from build123d import *

# Parameters (mm, degrees)
BOSS_EXTRUDE1_DEPTH = 50
SKETCH2_R           = 22.5
BOSS_EXTRUDE2_DEPTH = 20
SKETCH3_R           = 22.5
BOSS_EXTRUDE3_DEPTH = 20
CHAMFER2_SIZE       = 2


with BuildPart() as part:
    # Sketch1 → Boss-Extrude1 (new body)
    with BuildSketch(Plane.XY):
        Polygon((0, 275), (0, 0), (275, 0), (275, 15), (15, 15), (15, 275), align=None)
    extrude(amount=BOSS_EXTRUDE1_DEPTH)

    # Sketch2 → Boss-Extrude2 (add)
    with BuildSketch(Plane(origin=(0, 15, 0), x_dir=(1, 0, 0), z_dir=(0, 1, 0))):
        with Locations((145, -25)):
            Circle(SKETCH2_R)
    extrude(amount=BOSS_EXTRUDE2_DEPTH)

    # Sketch3 → Boss-Extrude3 (add)
    with BuildSketch(Plane(origin=(15, 0, 0), x_dir=(0, 0, -1), z_dir=(1, 0, 0))):
        with Locations(Location((-25, 145, 0), (0, 0, 180))):
            Circle(SKETCH3_R)
    extrude(amount=BOSS_EXTRUDE3_DEPTH)

    # Chamfer2
    chamfer2_edges = [part.edges().sort_by_distance(p)[0] for p in [
        (0, 0, 25),
        (0, 275, 25),
        (0, 137.5, 0),
        (0, 137.5, 50),
    ]]
    chamfer(chamfer2_edges, length=CHAMFER2_SIZE)


solid = part.part
CAD build for the part. Positions are in the model's coordinates, mm. A direction names the side the tool comes from. Give positions to 0.01 mm unless a question says otherwise; leave off trailing zeros. Loops run counter-clockwise (first coordinate to the right, second up) from the corner with the lowest first, then second, coordinate; pieces in that order, holes last. Notation, with made-up numbers: M -31,-4 L 14,-4 A30 ccw 14,35 Z; hole C 85.25,38 d11. An arc over 180 degrees is marked long. One line per question, with ' | ' between items. Start each with the question number.
1. Saw through at C-C on y = 145. Give the cut face in (x, z), plus the area to 3 significant figures.
2. Saw through at A-A on x = 145. Give the cut face in (y, z), plus the area to 3 significant figures.
3. 3-axis set-ups, long thin cutter, end or side, ignore diameter. For faces 1 (the face through (137, 0, 25)), 2 (the face through (166.46, 24.86, 18.24)), 3 (the face through (35, 145, 25)): which of +Z, -Z, +X, -X, +Y, -Y reach the whole face in a straight line?
4. Flat gauge pins, fed straight in: pin 1 (13.5 mm diameter, centred on x = 135.5, z = 19.5, fed in from +Y); pin 2 (22.5 mm diameter, centred on y = 137.5, z = 23.5, fed in from +X); pin 3 (12 mm diameter, centred on y = 74.5, z = 45, fed in from +X). Where does each tip first touch, or does it go through?
5. Two-plate mould, pull along X, no slides. Class faces 4 (the face through (147, 15, 2)), 5 (the face through (24.86, 122.69, 22.07)), 6 (the face through (0, 139, 25)): pulls with the +X half, pulls with the -X half, needs draft (parallel to the pull), parting line crosses it, or undercut.
6. Saw through at D-D on z = 6.5. Give the cut face in (x, y).
7. Probe L1, parallel to X at y = 167, z = 30.5; L2, parallel to Y at x = 160.5, z = 36. List the from-to ranges inside material, lowest first. Write a range as from..to.
8. Saw through at B-B on z = 25. Give the cut face in (x, y), plus the area to 3 significant figures.
Result sheet:
1) outline: M 0,2 L 2,0 L 15,0 L 15,2.5 L 35,2.5 L 35,47.5 L 15,47.5 L 15,50 L 2,50 L 0,48 Z | area: 1,650 mm^2
2) outline: M 0,0 L 15,0 L 15,2.5 L 35,2.5 L 35,47.5 L 15,47.5 L 15,50 L 0,50 Z | area: 1,650 mm^2
3) face 1: +Z, -Z, +X, -X, -Y | face 2: +Y | face 3: +Z, -Z, +X, +Y
4) pin 1: stops at y = 35 | pin 2: stops at x = 35 | pin 3: stops at x = 15
5) face 4: undercut | face 5: needs draft | face 6: pulls with the -X half
6) outline: M 0,2 L 2,0 L 275,0 L 275,15 L 157.81,15 L 157.81,35 L 132.19,35 L 132.19,15 L 15,15 L 15,132.19 L 35,132.19 L 35,157.81 L 15,157.81 L 15,275 L 2,275 L 0,273 Z
7) L1: x = 0..15 | L2: y = 0..35
8) outline: M 0,2 L 2,0 L 275,0 L 275,15 L 167.5,15 L 167.5,35 L 122.5,35 L 122.5,15 L 15,15 L 15,122.5 L 35,122.5 L 35,167.5 L 15,167.5 L 15,275 L 2,275 L 0,273 Z | area: 9,820 mm^2
